For this review, take the finished solid that the model builds, in its own axes (mm). Face numbers are marked on the shaded views. A direction names the side the tool comes from. Give positions to 0.01 mm unless a question says otherwise; leave off trailing zeros. Order: outer loops, then holes, each group sorted by start corner. A loop starts at its lowest first (then second) coordinate and runs counter-clockwise, first axis right, second up.
Item 1: The part is to be moulded in two halves that separate along Y. For the marked faces 3, 4 and 5, say which applies: released by +Y, released by -Y, zero draft, split by the parting line, or undercut.
Item 2: Consider section C-C (x = -13). Give the boundary of the cut face in (y, z), plus the area to 3 significant figures.
Item 3: For probe 1 along Z at (x, y) = (-14.25, 2.5); probe 2 along Y at (x, z) = (-13.25, 2.8); probe 3 along Y at (x, z) = (-11.25, 0.8), list the stretches that pass through material, from the lowest coordinate up.
Item 4: Consider section D-D (x = -10.25). Give the boundary of the cut face in (y, z), plus the area to 3 significant figures.
Item 5: Consider section A-A (y = -6.75). Give the boundary of the cut face in (x, z), plus the area to 3 significant figures.
Item 6: For P1, Ø3, axis at x = -15, y = 0.5, coming from the +Z side; P2, Ø4, axis at x = -12.79, y = -5.97, coming from the +Z side; P3, Ø2, axis at x = -13.5, z = 3.5, coming from the +Y side, all flat-tipped, find the tip position at first contact; note any pin that passes through.
Item 7: Consider section B-B (z = 0.7). Give the boundary of the cut face in (x, y), plus the area to 3 significant figures.
Item 8: Machinability: for the marked faces 1 and 2, which of the approach directions +Z, -Z, +X, -X, +Y, -Y give a long, thin tool a straight path to every point of the face, cutting with its end or side? Answer none if there is none.
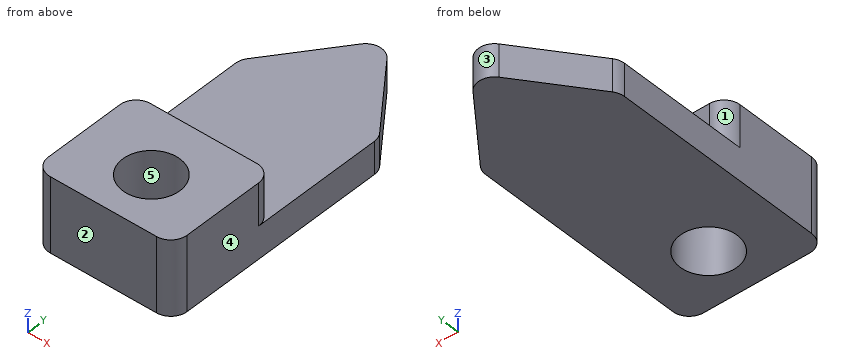
```python
from build123d import *

# Parameters (mm, degrees)
F0_R     = 1.75
F1_DEPTH = 4.6
F2_DEPTH = 2
F3_R     = 1
F4_R     = 1
F5_R     = 1
F6_R     = 1


with BuildPart() as f1:
    # F0 (on Top) → F1 (new body)
    with BuildSketch(Plane.XY):
        Polygon((-17.207691, -2.142988), (-17.207691, -9.142705), (-8.686733, -9.142705), (-8.686733, -2.142988), (-16.240229, -2.142988), align=None)
        with Locations((-12.791907, -5.968139)):
            Circle(F0_R, mode=Mode.SUBTRACT)
    extrude(amount=F1_DEPTH)

    # F0 (on Top) → F2 (join)
    with BuildSketch(Plane.XY):
        Polygon((-17.207691, 5.29756), (-17.207691, -2.142988), (-16.240229, -2.142988), (-8.686733, -2.142988), (-8.686733, 5.29756), (-12.975041, 10.857295), align=None)
    extrude(amount=F2_DEPTH)

    # F3
    f3_edges = [f1.edges().sort_by_distance(p)[0] for p in [
        (-8.686733, -9.142705, 2.3),
    ]]
    fillet(f3_edges, radius=F3_R)

    # F4
    f4_edges = [f1.edges().sort_by_distance(p)[0] for p in [
        (-17.207691, -9.142705, 2.3),
    ]]
    fillet(f4_edges, radius=F4_R)

    # F5
    f5_edges = [f1.edges().sort_by_distance(p)[0] for p in [
        (-17.207691, -2.142988, 3.3),
    ]]
    fillet(f5_edges, radius=F5_R)

    # F6
    f6_edges = [f1.edges().sort_by_distance(p)[0] for p in [
        (-8.686733, -2.142988, 3.3),
        (-12.975041, 10.857295, 1),
        (-8.686733, 5.29756, 1),
        (-17.207691, 5.29756, 1),
    ]]
    fillet(f6_edges, radius=F6_R)


solid = f1.part
```
Resolved:
1. face 3: released by +Y
1. face 4: zero draft
1. face 5: undercut
2. outline: (-9.14, 0) - (-7.71, 0) - (-7.71, 4.6) - (-9.14, 4.6) - close; (-4.23, 0) - (10.21, 0) - (10.21, 2) - (-2.14, 2) - (-2.14, 4.6) - (-4.23, 4.6) - close
2. area: 40.9 mm2
3. probe 1: z = 0 to 2
3. probe 2: y = -9.14 to -7.66, -4.28 to -2.14
3. probe 3: y = -9.14 to -6.8, -5.14 to 8.62
4. outline: (-9.14, 0) - (7.32, 0) - (7.32, 2) - (-2.14, 2) - (-2.14, 4.6) - (-9.14, 4.6) - close
4. area: 51.1 mm2
5. outline: (-17.21, 0) - (-14.36, 0) - (-14.36, 4.6) - (-17.21, 4.6) - close; (-11.23, 0) - (-8.69, 0) - (-8.69, 4.6) - (-11.23, 4.6) - close
5. area: 24.8 mm2
6. P1: stops at z = 2
6. P2: stops at z = 4.6
6. P3: stops at y = -2.14
7. outline: (-17.21, -8.14) arc R1 ccw to (-16.21, -9.14) - (-9.69, -9.14) arc R1 ccw to (-8.69, -8.14) - (-8.69, 4.96) arc R1 ccw to (-8.89, 5.57) - (-12.18, 9.82) arc R1 ccw to (-13.77, 9.82) - (-17, 5.57) arc R1 ccw to (-17.21, 4.96) - close; hole circle Ø3.5 at (-12.79, -5.97)
7. area: 136 mm2
8. face 1: +Z, -X, +Y
8. face 2: +Z, -Z, +X, -X, -Y
